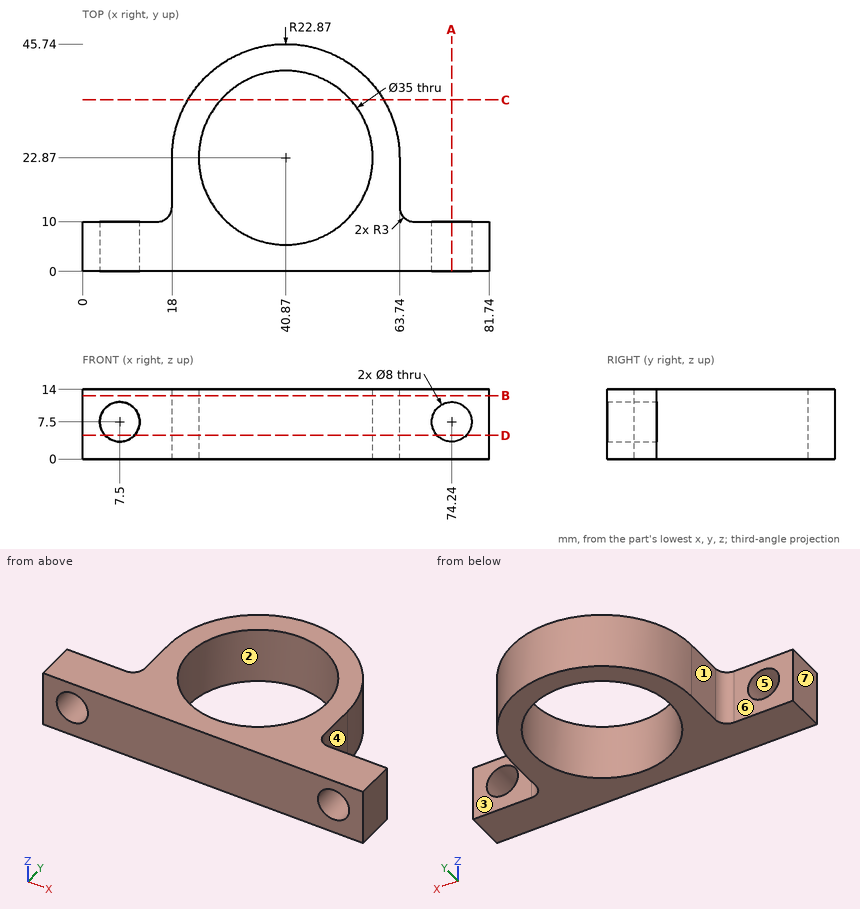
Design review of the part shown in the three views and the two pictorial views. Dimensions are in mm from the part's minimum x, y and z. A direction names the side the tool comes from. Round coordinates to 2 decimals unless told otherwise and drop trailing zeros. Loops run counter-clockwise (first coordinate to the right, second up) from the corner with the lowest first, then second, coordinate; pieces in that order, holes last. Notation, with made-up numbers: M 60.5,41 L 118.5,41 A12 ccw 118.5,50 Z; hole C 16,-10 d8. An arc over 180 degrees is marked long. Put each result on its own line as item: value.
Q1. Consider section D-D, the plane z = 4.75. Give the boundary of the cut face in (x, y), then the cut area to 3 significant figures.
Result set:
outline: M 0,0 L 4.6,0 L 4.6,10 L 0,10 Z; M 10.4,0 L 71.34,0 L 71.34,10 L 66.74,10 A3 cw 63.74,13 L 63.74,22.87 A22.87 ccw 18,22.87 L 18,13 A3 cw 15,10 L 10.4,10 Z; M 77.14,0 L 81.74,0 L 81.74,10 L 77.14,10 Z; hole C 40.87,22.87 d35
area: 1,150 mm²
Q2. Consider section C-C, the plane y = 34.5. Give the boundary of the cut face in (x, z).
Result set:
outline: M 21.18,0 L 27.79,0 L 27.79,14 L 21.18,14 Z; M 53.95,0 L 60.56,0 L 60.56,14 L 53.95,14 Z
Q3. For pin 1 (4 mm diameter, centred on x = 48, z = 5.5, fed in from +Y); pin 2 (1 mm diameter, centred on x = 63.5, y = 20.5, fed in from -Z); pin 3 (8 mm diameter, centred on x = 57.5, z = 11, fed in from +Y); pin 4 (6.5 mm diameter, centred on x = 74.24, z = 7.5, fed in from +Y), all flat-tipped, find the tip position at first contact; note any pin that passes through.
Result set:
pin 1: stops at y = 45.16
pin 2: stops at z = 0
pin 3: stops at y = 41.94
pin 4: passes through
Q4. Consider section A-A, the plane x = 74.24. Give the boundary of the cut face in (y, z), then the cut area to 3 significant figures.
Result set:
outline: M 0,0 L 10,0 L 10,3.5 L 0,3.5 Z; M 0,11.5 L 10,11.5 L 10,14 L 0,14 Z
area: 60.0 mm²
Q5. Mouldability with a two-part tool opening along X and no side actions: class the marked faces 4, 5, 6 and 7 as released by +X, released by -X, zero draft, split by the parting line, or undercut.
Result set:
face 4: released by +X
face 5: undercut
face 6: zero draft
face 7: released by -X
Q6. Consider section B-B, the plane z = 12.75. Give the boundary of the cut face in (x, y), then the cut area to 3 significant figures.
Result set:
outline: M 0,0 L 81.74,0 L 81.74,10 L 66.74,10 A3 cw 63.74,13 L 63.74,22.87 A22.87 ccw 18,22.87 L 18,13 A3 cw 15,10 L 0,10 Z; hole C 40.87,22.87 d35
area: 1,270 mm²
Q7. To check wall thickness, follow L1, parallel to X at y = 3.75, z = 7.5; L2, parallel to Z at x = 74.24, y = 6; L3, parallel to Y at x = 40.87, z = 6. State the ranges of each line that lie inside material, in increasing order.
Result set:
L1: x = 0 to 3.5, 11.5 to 70.24, 78.24 to 81.74
L2: z = 0 to 3.5, 11.5 to 14
L3: y = 0 to 5.37, 40.37 to 45.74
Q8. Machinability: for the marked faces 1, 2 and 3, which of the approach directions +Z, -Z, +X, -X, +Y, -Y give a long, thin tool a straight path to every point of the face, cutting with its end or side? Answer none if there is none.
Result set:
face 1: +Z, -Z, -X, +Y
face 2: +Z, -Z
face 3: +Z, -Z, +X, +Y
